Model file for the job. Use its own axes, mm. A direction names the side the tool comes from. Give positions to 0.01 mm unless a question says otherwise; leave off trailing zeros. Order: outer loops, then holes, each group sorted by start corner. A loop starts at its lowest first (then second) coordinate and runs counter-clockwise, first axis right, second up. Notation, with made-up numbers: (-9, -16) -> (25, -16) arc R23 ccw to (25, 19) -> close; hole circle Ø8 at (74, 61). An arc over 180 degrees is marked (long way). Use CSV: the item, a comma, the result in double quotes. Start each with the question number.
1. Drop flat-ended pins along their axis: pin 1 (8 mm diameter, centred on x = 35, y = 22.5, fed in from +Z); pin 2 (21 mm diameter, centred on x = 0, y = 31.2, fed in from +Z); pin 3 (6 mm diameter, centred on y = 24, z = 20.5, fed in from -X); pin 4 (1 mm diameter, centred on x = -8, z = 25, fed in from +Y). Give the stop position or say it passes through.
2. Cut at C-C on z = 11. List the corners of the cut face in (x, y).
3. 3-axis set-ups, long thin cutter, end or side, ignore diameter. For faces 4 (the flat face through (-49.15, -16.04, 6.7)), 5 (the cylindrical face through (32.178, 19.555, 2.028)): which of +Z, -Z, +X, -X, +Y, -Y reach the whole face in a straight line?
4. Pull direction X, two halves, no side cores. Call faces 1 (the flat face through (-1, 1, 0)), 2 (the cylindrical face through (-11.164, -50.275, 22.644)), 3 (the flat face through (-1, 1, 4)): released by +X, released by -X, zero draft, split by the parting line, or undercut.
5. Cut at B-B on x = 0. Give the number of separate pieces and of enclosed holes in the cut face, then the cut area to 3 significant figures.
6. Cut at A-A on y = 0. List the corners of the cut face in (x, z), then the cut area to 3 significant figures.
7. Wall check: line 1 (Y direction, x = 0, z = 1.4); line 2 (X direction, y = -15, z = 3); line 3 (Z direction, x = -24, y = 28). Give the ranges that are in metal, low to high. Write a range as from..to.
```python
from build123d import *

# Parameters (mm, degrees)
CROQUIS1_R                    = 55
SALIENTE_EXTRUIR1_DEPTH       = 6.7
CROQUIS2_R                    = 51.5
SALIENTE_EXTRUIR2_DEPTH       = 30
CROQUIS3_R                    = 2
CROQUIS4_R                    = 43.2
CORTAR_EXTRUIR1_DEPTH         = 32.7
TALADRO_DE_MARGEN_PARA_M121_D = 13
MATRIZC1_COUNT                = 6
TALADRO_DE_MARGEN_PARA_M122_D = 13


with BuildPart() as part:
    # Croquis1 → Saliente-Extruir1 (new body)
    with BuildSketch(Plane.XY):
        Circle(CROQUIS1_R)
    extrude(amount=SALIENTE_EXTRUIR1_DEPTH)

    # Croquis2 → Saliente-Extruir2 (add)
    with BuildSketch(Plane.XY.offset(6.7)):
        Circle(CROQUIS2_R)
    extrude(amount=SALIENTE_EXTRUIR2_DEPTH)

    # Croquis3 → Cortar-Revolución1 (revolve, cut)
    with BuildSketch(Plane(origin=(0, 0, 0), x_dir=(1, 0, 0), z_dir=(0, 1, 0)), mode=Mode.PRIVATE) as cortar_revoluci_n1_sk:
        with Locations((-51.5, -16.7)):
            Circle(CROQUIS3_R)
        with Locations((-51.5, -28.7)):
            Circle(CROQUIS3_R)
    revolve(cortar_revoluci_n1_sk.sketch.rotate(Axis((0, 0, 36.878025431), (0, 0, -1)), 180), axis=Axis((0, 0, 36.878025431), (0, 0, -1)), mode=Mode.SUBTRACT)

    # Croquis4 → Cortar-Extruir1 (cut)
    with BuildSketch(Plane.XY.offset(36.7)):
        Circle(CROQUIS4_R)
    extrude(amount=-CORTAR_EXTRUIR1_DEPTH, mode=Mode.SUBTRACT)

    # Taladro de margen para M121 (through all)
    with Locations(Plane(origin=(0, 0, 0), x_dir=(-1, 0, 0), z_dir=(0, 0, -1))):
        with Locations((0, 31.2)):
            taladro_de_margen_para_m121 = Hole(TALADRO_DE_MARGEN_PARA_M121_D / 2)

    # MatrizC1: Taladro de margen para M121 ×6 about axis
    matrizc1_axis = Axis((0, 0, 0), (0, 0, 1))
    for i in range(1, MATRIZC1_COUNT):
        add(taladro_de_margen_para_m121.rotate(matrizc1_axis, i * 360 / MATRIZC1_COUNT), mode=Mode.SUBTRACT)

    # Taladro de margen para M122 (through all)
    with Locations(Plane(origin=(0, 0, 0), x_dir=(-1, 0, 0), z_dir=(0, 0, -1))):
        with Locations((0, -9.6)):
            taladro_de_margen_para_m122 = Hole(TALADRO_DE_MARGEN_PARA_M122_D / 2)

    # Simetría1: Taladro de margen para M122 across plane
    add(taladro_de_margen_para_m122.mirror(Plane.ZX), mode=Mode.SUBTRACT)


solid = part.part
```
Verdict:
1,pin 1,"z = 36.7"
1,pin 2,"z = 4"
1,pin 3,"x = -47.02"
1,pin 4,"y = 50.95"
2,outline,"circle Ø103 at (0, 0); hole circle Ø86.4 at (0, 0)"
3,face 4,"+Z"
3,face 5,"+Z, -Z"
4,face 1,"zero draft"
4,face 2,"split by the parting line"
4,face 3,"undercut"
5,separate pieces,"5"
5,enclosed holes,"0"
5,area,"769 mm^2"
6,outline,"(-55, 0) -> (55, 0) -> (55, 6.7) -> (51.5, 6.7) -> (51.5, 14.7) arc R2 cw to (51.5, 18.7) -> (51.5, 26.7) arc R2 cw to (51.5, 30.7) -> (51.5, 36.7) -> (43.2, 36.7) -> (43.2, 4) -> (-43.2, 4) -> (-43.2, 36.7) -> (-51.5, 36.7) -> (-51.5, 30.7) arc R2 cw to (-51.5, 26.7) -> (-51.5, 18.7) arc R2 cw to (-51.5, 14.7) -> (-51.5, 6.7) -> (-55, 6.7) -> close"
6,area,"977 mm^2"
7,line 1,"-55..-37.7, -24.7..-16.1, -3.1..3.1, 16.1..24.7, 37.7..55"
7,line 2,"-52.92..-33.49, -20.55..-3.62, 3.62..20.55, 33.49..52.92"
7,line 3,"0..4"
